from build123d import *

# Parameters (mm, degrees)
F1_DEPTH      = 7.62
F0_R          = 16.67939
F2_DEPTH      = 25.4
F4_DEPTH      = 7.62
F4_DEPTH_BACK = 7.62


with BuildPart() as f1:
    # F0 (on Top) → F1 (new body)
    with BuildSketch(Plane.XY):
        with BuildLine():
            Line((22.05117, -16.240392), (22.05117, 37.099611))
            ThreePointArc((22.05117, 37.099611), (0, 15.048441), (-22.05117, 37.099611))
            Line((-22.05117, 37.099611), (-22.05117, -16.240392))
            Line((-22.05117, -16.240392), (22.05117, -16.240392))
        make_face()
    extrude(amount=F1_DEPTH)

    # F0 (on Top) → F2 (join)
    with BuildSketch(Plane.XY):
        with BuildLine():
            ThreePointArc((-22.05117, 37.099611), (0, 15.048441), (22.05117, 37.099611))
            ThreePointArc((22.05117, 37.099611), (0, 59.150781), (-22.05117, 37.099611))
        make_face()
        with Locations((0, 37.099611)):
            Circle(F0_R, mode=Mode.SUBTRACT)
    extrude(amount=F2_DEPTH)

    # F3 (on Right) → F4 (join, two sides)
    with BuildSketch(Plane.YZ) as f4_sk:
        Polygon((15.197432, 23.466621), (0, 7.62), (15.197432, 7.62), align=None)
    extrude(amount=F4_DEPTH)
    extrude(f4_sk.sketch, amount=-F4_DEPTH_BACK)


solid = f1.part
The model under review builds one solid part; all positions refer to its coordinate system, in mm. A direction names the side the tool comes from. Coordinates: 2 decimals unless noted, no trailing zeros. Write each loop counter-clockwise with the first axis right and the second up, starting at its lowest first coordinate (ties: lowest second). Pieces come first, ordered by that corner, then holes. Notation, with made-up numbers: (26.25, 29.25) - (74.25, 29.25) arc R30 ccw to (74.25, 52.25) - close; hole circle Ø2 at (-7, 40.5). An arc over 180 degrees is marked (long way). Answer as CSV lines item,"result".
(1) Clearance check with flat-ended pins moving along their axes: pin 1 Ø8 at (x, z) = (15, 11) entering from +Y; pin 2 Ø12 at (y, z) = (17.5, 18.5) entering from +X; pin 3 Ø5.5 at (x, z) = (5.5, 19.5) entering from +Y. State where each tip first meets the part, or that it passes through.
Data:
pin 1,"stops at y = 56.21"
pin 2,"stops at x = 17.36"
pin 3,"stops at y = 58.98"
(2) We need section B-B (x = 0). Give the boundary of the cut face in (y, z), plus the area to 3 significant figures.
Data:
outline,"(-16.24, 0) - (20.42, 0) - (20.42, 25.4) - (15.05, 25.4) - (15.05, 23.31) - (0, 7.62) - (-16.24, 7.62) - close; (53.78, 0) - (59.15, 0) - (59.15, 25.4) - (53.78, 25.4) - close"
area,"629 mm2"
(3) Mouldability with a two-part tool opening along Y and no side actions: class faces 4 (the flat face through (0, -16.24, 4)), 5 (the flat face through (-5, 15.197, 15)), 6 (the flat face through (0, 14, 0)) as pulls with the +Y half, pulls with the -Y half, needs draft (parallel to the pull), parting line crosses it, or undercut.
Data:
face 4,"pulls with the -Y half"
face 5,"undercut"
face 6,"needs draft"
(4) For line 1 along Z through (x, y) = (19.5, -8); line 2 along Y through (x, z) = (0, 18.5); line 3 along Y through (x, z) = (9.5, 4.5), list the stretches that pass through material, from the lowest coordinate up. Write a range as [from, to].
Data:
line 1,"z = [0, 7.62]"
line 2,"y = [10.43, 20.42], [53.78, 59.15]"
line 3,"y = [-16.24, 23.39], [50.81, 57]"
(5) We need section D-D (y = 39.5). Give the boundary of the cut face in (x, z), plus the area to 3 significant figures.
Data:
outline,"(-21.92, 0) - (-16.51, 0) - (-16.51, 25.4) - (-21.92, 25.4) - close; (16.51, 0) - (21.92, 0) - (21.92, 25.4) - (16.51, 25.4) - close"
area,"275 mm2"
(6) We need section C-C (z = 2.5). Give the boundary of the cut face in (x, y), plus the area to 3 significant figures.
Data:
outline,"(-22.05, -16.24) - (22.05, -16.24) - (22.05, 37.1) arc R22.05 ccw to (-22.05, 37.1) - close; hole circle Ø33.36 at (0, 37.1)"
area,"2,240 mm2"
(7) Tool access review of faces 1 (the flat face through (7.62, 11, 12)), 2 (the flat face through (-7.62, 11, 12)), 3 (the flat face through (-22.051, 11, 4)): name each direction out of +Z, -Z, +X, -X, +Y, -Y from which nothing blocks a thin tool from reaching the whole face with its end or side.
Data:
face 1,"+Z, +X, -Y"
face 2,"+Z, -X, -Y"
face 3,"+Z, -Z, -X, +Y, -Y"
(8) We need section A-A (y = 28). Give the boundary of the cut face in (x, z).
Data:
outline,"(-22.05, 0) - (-13.98, 0) - (-13.98, 25.4) - (-20.09, 25.4) - (-20.09, 7.62) - (-22.05, 7.62) - close; (13.98, 0) - (22.05, 0) - (22.05, 7.62) - (20.09, 7.62) - (20.09, 25.4) - (13.98, 25.4) - close"
